```python
from build123d import *

# Parameters (mm, degrees)
SKETCH1_W                = 30
SKETCH1_H                = 2
BOSS_EXTRUDE2_DEPTH      = 0.5
SKETCH2_W                = 27.5
SKETCH2_H                = 2
BOSS_EXTRUDE4_DEPTH      = 0.75
BOSS_EXTRUDE4_DEPTH_BACK = 1.25
SKETCH3_W                = 1.25
SKETCH3_H                = 0.5
BOSS_EXTRUDE5_DEPTH      = 5
SKETCH4_W                = 1.25
SKETCH4_H                = 0.5
BOSS_EXTRUDE6_DEPTH      = 5


with BuildPart() as part:
    # Sketch1 → Boss-Extrude2 (new body)
    with BuildSketch(Plane.XY):
        with Locations((15, 1)):
            Rectangle(SKETCH1_W, SKETCH1_H)
    extrude(amount=BOSS_EXTRUDE2_DEPTH)

    # Sketch2 → Boss-Extrude4 (add, two sides)
    with BuildSketch(Plane.XY.offset(0.5)) as boss_extrude4_sk:
        with Locations((15, 1)):
            Rectangle(SKETCH2_W, SKETCH2_H)
    extrude(amount=BOSS_EXTRUDE4_DEPTH)
    extrude(boss_extrude4_sk.sketch, amount=-BOSS_EXTRUDE4_DEPTH_BACK)

    # Sketch3 → Boss-Extrude5 (add)
    with BuildSketch(Plane.XZ):
        with Locations((0.625, 0.25)):
            Rectangle(SKETCH3_W, SKETCH3_H)
    extrude(amount=BOSS_EXTRUDE5_DEPTH)

    # Sketch4 → Boss-Extrude6 (add)
    with BuildSketch(Plane(origin=(0, 0, 0), x_dir=(-1, 0, 0), z_dir=(0, -1, 0))):
        with Locations((-29.375, -0.25)):
            Rectangle(SKETCH4_W, SKETCH4_H)
    extrude(amount=BOSS_EXTRUDE6_DEPTH)


solid = part.part
```
Here's how the part is built. I have some questions about the finished solid (model axes, mm). A direction names the side the tool comes from. Give positions to 0.01 mm unless a question says otherwise; leave off trailing zeros. Order: outer loops, then holes, each group sorted by start corner. A loop starts at its lowest first (then second) coordinate and runs counter-clockwise, first axis right, second up. Notation, with made-up numbers: M -21.75,56 L 29.25,56 A27 ccw 29.25,79 Z; hole C -17,69 d8. An arc over 180 degrees is marked long. Use a Markdown table: item, result. Add a question column.
1. On a 3-axis mill with a long thin cutter (end or side, diameter ignored), from which of +Z, -Z, +X, -X, +Y, -Y can I reach the whole of each face in a straight line? I mean faces 1 (the flat face through (29, -1, 0.5)), 2 (the flat face through (29, -1, 0)), 3 (the flat face through (15, 1, 1.25)), 4 (the flat face through (1, -1, 0)), 5 (the flat face through (15, 2, 0)). Say none if no direction works.
2. If we mould it in two halves opening along X, with no side actions, what happens to faces 6 (the flat face through (1, -1, 0.5)), 7 (the flat face through (15, 0, 0))? For each: +X half, -X half, draft (parallel to the pull), parting line (faces both ways), or undercut.
3. Suppose I cut it at D-D (z = -0.4). List the corners of the cut face in (x, y) for me, and give its area (3 significant figures).
4. Suppose I cut it at B-B (y = 1). List the corners of the cut face in (x, z) for me, and give its area (4 significant figures).
5. Suppose I cut it at A-A (y = -2.5). List the corners of the cut face in (x, z) for me.
6. Suppose I cut it at C-C (x = 2.25). List the corners of the cut face in (y, z) for me.
7. For pin 1 Ø1.4 at (x, y) = (0.5, -3) entering from -Z; pin 2 Ø0.6 at (y, z) = (1, -0.5) entering from +X; pin 3 Ø1.4 at (x, y) = (29, -1.5) entering from +Z; pin 4 Ø2 at (x, y) = (9.5, -1.5) entering from -Z, each with a flat end and sliding along its axis, tell me the tip position at first contact or that it passes through.
8. I need wall thicknesses on probe 1 along X at (y, z) = (1.25, 0.75); probe 2 along X at (y, z) = (-1.25, 0.15); probe 3 along Y at (x, z) = (10, 0.35). Which ranges of each line are inside material? Lowest first, please. Write a range as from..to.
Results list:
| question | item | result |
|---|---|---|
| 1 | face 1 | +Z, +X, +Y, -Y |
| 1 | face 2 | -Z, +X, +Y, -Y |
| 1 | face 3 | +Z, +X, -X, +Y, -Y |
| 1 | face 4 | -Z, -X, +Y, -Y |
| 1 | face 5 | +Z, -Z, +X, -X, +Y |
| 2 | face 6 | draft |
| 2 | face 7 | undercut |
| 3 | outline | M 1.25,0 L 28.75,0 L 28.75,2 L 1.25,2 Z |
| 3 | area | 55.0 mm² |
| 4 | outline | M 0,0 L 1.25,0 L 1.25,-0.75 L 28.75,-0.75 L 28.75,0 L 30,0 L 30,0.5 L 28.75,0.5 L 28.75,1.25 L 1.25,1.25 L 1.25,0.5 L 0,0.5 Z |
| 4 | area | 56.25 mm² |
| 5 | outline | M 0,0 L 1.25,0 L 1.25,0.5 L 0,0.5 Z; M 28.75,0 L 30,0 L 30,0.5 L 28.75,0.5 Z |
| 6 | outline | M 0,-0.75 L 2,-0.75 L 2,1.25 L 0,1.25 Z |
| 7 | pin 1 | stops at z = 0 |
| 7 | pin 2 | stops at x = 28.75 |
| 7 | pin 3 | stops at z = 0.5 |
| 7 | pin 4 | passes through |
| 8 | probe 1 | x = 1.25..28.75 |
| 8 | probe 2 | x = 0..1.25, 28.75..30 |
| 8 | probe 3 | y = 0..2 |
